Part model, mm, in its own coordinate system. A direction names the side the tool comes from. Round coordinates to 2 decimals unless told otherwise and drop trailing zeros. Loops run counter-clockwise (first coordinate to the right, second up) from the corner with the lowest first, then second, coordinate; pieces in that order, holes last.
1) Probe line 1 (Z direction, x = -9, y = 14); line 2 (X direction, y = 8.5, z = 3); line 3 (X direction, y = 33.96, z = 10.75). List the from-to ranges inside material, lowest first.
2) Band-saw the part on A-A, the plane y = 33.96. Write the cut outline in (x, z), then the cut area to 3 significant figures.
3) Band-saw the part on C-C, the plane z = 4. Write the cut outline in (x, y), then the cut area to 3 significant figures.
4) Mould opens along X. For faces 1 (the flat face through (0, -47.5, 8)), 2 (the flat face through (0, -44.5, 6)), 3 (the flat face through (-30.744, -0.714, -1.514)) say: +X half, -X half, draft (parallel to the pull), parting line (faces both ways), or undercut.
5) Band-saw the part on B-B, the plane x = 19. Write the cut outline in (y, z), then the cut area to 3 significant figures.
6) 3-axis set-ups, long thin cutter, end or side, ignore diameter. For faces 4 (the flat face through (-22, 35, 8)), 5 (the cylindrical face through (-0.283, 47.497, 8.381)), 6 (the flat face through (-30.25, -7, 8)), 7 (the flat face through (30.25, -6, 8)), 8 (the flat face through (-19, 32, 6)): which of +Z, -Z, +X, -X, +Y, -Y reach the whole face in a straight line?
7) Drop flat-ended pins along their axis: P1, Ø6, axis at x = -19, z = -4, coming from the -Y side; P2, Ø13.5, axis at x = -13.5, z = 12, coming from the -Y side; P3, Ø5, axis at y = -29, z = -4, coming from the +X side. Give the stop position or say it passes through.
from build123d import *
from OCP.BRepFilletAPI import BRepFilletAPI_MakeChamfer

# Parameters (mm, degrees)
BOSS_EXTRUDE1_DEPTH = 17
SKETCH2_W           = 65
SKETCH2_H           = 102
BOSS_EXTRUDE2_DEPTH = 2.5
SHELL1_START        = -2.5
SHELL1_DEPTH        = 16.5
CHAMFER1_SIZE       = 2
CHAMFER1_SIZE2      = 3.464101615
SKETCH3_W           = 56.07179677
SKETCH3_H           = 93.07179677
BOSS_EXTRUDE3_DEPTH = 1
SKETCH5_R           = 7.637477526
BOSS_EXTRUDE4_DEPTH = 10
BOSS_EXTRUDE4_TAPER = 2
FILLET1_R           = 2


# Read off the part's stored shape, not the designer's step: Shell1
with BuildPart() as part:
    # Sketch1 → Boss-Extrude1 (new body)
    with BuildSketch(Plane.XY):
        with BuildLine():
            Line((13.5, 35), (30.25, 35))
            Line((30.25, 35), (30.25, -47.5))
            Line((30.25, -47.5), (-30.25, -47.5))
            Line((-30.25, -47.5), (-30.25, 35))
            Line((-30.25, 35), (-13.5, 35))
            ThreePointArc((-13.5, 35), (0, 47.5), (13.5, 35))
        make_face()
    extrude(amount=BOSS_EXTRUDE1_DEPTH)

    # Sketch2 → Boss-Extrude2 (add)
    with BuildSketch(Plane(origin=(0, 0, 0), x_dir=(-1, 0, 0), z_dir=(0, 0, -1))):
        Rectangle(SKETCH2_W, SKETCH2_H)
    extrude(amount=BOSS_EXTRUDE2_DEPTH)

    # Shell1 outline → Shell1 (cut)
    with BuildSketch(Plane.XY.offset(SHELL1_START)):
        with BuildLine():
            Line((27.25, -44.5), (27.25, 32))
            Line((27.25, 32), (10.356157589, 32))
            ThreePointArc((10.356157589, 32), (0, 44.5), (-10.356157589, 32))
            Line((-10.356157589, 32), (-27.25, 32))
            Line((-27.25, 32), (-27.25, -44.5))
            Line((-27.25, -44.5), (27.25, -44.5))
        make_face()
    extrude(amount=SHELL1_DEPTH, mode=Mode.SUBTRACT)

    # Chamfer1: one chamfer whose edges measure the first distance from different faces: ONE call of the kernel's chamfer builder (chamfer() names one face for all edges)
    chamfer1_edges_1 = [part.edges().sort_by_distance(p)[0] for p in [
        (0, -51, -2.5),
    ]]
    chamfer1_side_1 = [part.faces().sort_by_distance(p)[0] for p in [
        (0, -51, -1.25),
    ]]
    chamfer1_edges_2 = [part.edges().sort_by_distance(p)[0] for p in [
        (32.5, 0, -2.5),
    ]]
    chamfer1_side_2 = [part.faces().sort_by_distance(p)[0] for p in [
        (32.5, 0, -1.25),
    ]]
    chamfer1_edges_3 = [part.edges().sort_by_distance(p)[0] for p in [
        (0, 51, -2.5),
    ]]
    chamfer1_side_3 = [part.faces().sort_by_distance(p)[0] for p in [
        (0, 51, -1.25),
    ]]
    chamfer1_edges_4 = [part.edges().sort_by_distance(p)[0] for p in [
        (-32.5, 0, -2.5),
    ]]
    chamfer1_side_4 = [part.faces().sort_by_distance(p)[0] for p in [
        (-32.5, 0, -1.25),
    ]]
    chamfer1 = BRepFilletAPI_MakeChamfer(part.part.solid().wrapped)
    for e in chamfer1_edges_1:
        chamfer1.Add(CHAMFER1_SIZE, CHAMFER1_SIZE2, e.wrapped, chamfer1_side_1[0].wrapped)  # the first distance lies on this face
    for e in chamfer1_edges_2:
        chamfer1.Add(CHAMFER1_SIZE, CHAMFER1_SIZE2, e.wrapped, chamfer1_side_2[0].wrapped)  # the first distance lies on this face
    for e in chamfer1_edges_3:
        chamfer1.Add(CHAMFER1_SIZE, CHAMFER1_SIZE2, e.wrapped, chamfer1_side_3[0].wrapped)  # the first distance lies on this face
    for e in chamfer1_edges_4:
        chamfer1.Add(CHAMFER1_SIZE, CHAMFER1_SIZE2, e.wrapped, chamfer1_side_4[0].wrapped)  # the first distance lies on this face
    add(Compound.cast(chamfer1.Shape()), mode=Mode.REPLACE)

    # Sketch3 → Boss-Extrude3 (add)
    with BuildSketch(Plane(origin=(0, 0, -2.5), x_dir=(-1, 0, 0), z_dir=(0, 0, -1))):
        Rectangle(SKETCH3_W, SKETCH3_H)
    extrude(amount=BOSS_EXTRUDE3_DEPTH)

    # Sketch5 → Boss-Extrude4 (add)
    with BuildSketch(Plane(origin=(0, 0, -3.5), x_dir=(-1, 0, 0), z_dir=(0, 0, -1))):
        with Locations((18.314549778, 1.094735509)):
            Circle(SKETCH5_R)
    extrude(amount=BOSS_EXTRUDE4_DEPTH, taper=BOSS_EXTRUDE4_TAPER)

    # Fillet1
    fillet1_edges = [part.edges().sort_by_distance(p)[0] for p in [
        (-11.026279948, 1.094735509, -13.5),
    ]]
    fillet(fillet1_edges, radius=FILLET1_R)


solid = part.part
Reported:
1. line 1: z = -3.5 to -2.5, 14 to 17
1. line 2: x = -30.25 to -27.25, 27.25 to 30.25
1. line 3: x = -30.25 to -10.54, 10.54 to 30.25
2. outline: (-32.5, -0.5) - (-29.04, -2.5) - (-28.04, -2.5) - (-28.04, -3.5) - (28.04, -3.5) - (28.04, -2.5) - (29.04, -2.5) - (32.5, -0.5) - (32.5, 0) - (30.25, 0) - (30.25, 17) - (-30.25, 17) - (-30.25, 0) - (-32.5, 0) - close; hole (-10.54, -2.5) - (10.54, -2.5) - (10.54, 14) - (-10.54, 14) - close
2. area: 892 mm2
3. outline: (-30.25, -47.5) - (30.25, -47.5) - (30.25, 35) - (13.5, 35) arc R13.54 ccw to (-13.5, 35) - (-30.25, 35) - close; hole (-27.25, -44.5) - (27.25, -44.5) - (27.25, 32) - (10.36, 32) arc R10.54 ccw (long way) to (-10.36, 32) - (-27.25, 32) - close
3. area: 866 mm2
4. face 1: draft
4. face 2: undercut
4. face 3: -X half
5. outline: (-51, -0.5) - (-47.54, -2.5) - (-46.54, -2.5) - (-46.54, -3.5) - (46.54, -3.5) - (46.54, -2.5) - (47.54, -2.5) - (51, -0.5) - (51, 0) - (35, 0) - (35, 17) - (-47.5, 17) - (-47.5, 0) - (-51, 0) - close; hole (-44.5, -2.5) - (32, -2.5) - (32, 14) - (-44.5, 14) - close
5. area: 481 mm2
6. face 4: +Z, -X, +Y
6. face 5: +Z, +Y
6. face 6: +Z, -X, +Y, -Y
6. face 7: +Z, +X, +Y, -Y
6. face 8: none
7. P1: stops at y = -50.13
7. P2: stops at y = -47.5
7. P3: stops at x = 30.77
